Input: part model. Units: mm. Frame: model coordinates. Face numbers are marked on the shaded views. A direction names the side the tool comes from. Give positions to 0.01 mm unless a question says otherwise; leave off trailing zeros. Loops run counter-clockwise (first coordinate to the right, second up) from the corner with the lowest first, then second, coordinate; pieces in that order, holes last. Notation, with made-up numbers: (77.25, 62) -> (111.25, 62) arc R17 cw to (111.25, 82) -> close; hole circle Ø9 at (53, 76.25). An arc over 180 degrees is marked (long way). One line per question, with ' | ' between items.
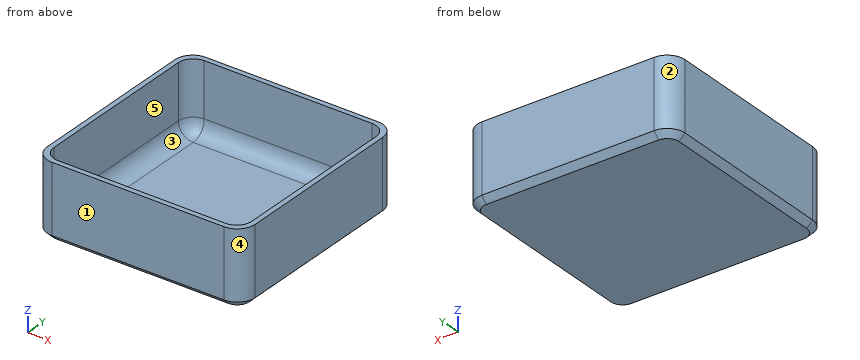
from build123d import *

# Parameters (mm, degrees)
F0_W     = 70
F0_H     = 70
F0_W_2   = 66.6
F0_H_2   = 66.6
F1_DEPTH = 25
F2_W     = 66.6
F2_H     = 66.6
F3_DEPTH = 23.3
F4_R     = 5
F5_R     = 6
F6_SIZE  = 2


with BuildPart() as f1:
    # F0 (on Top) → F1 (new body)
    with BuildSketch(Plane.XY):
        Rectangle(F0_W, F0_H)
        Rectangle(F0_W_2, F0_H_2, mode=Mode.SUBTRACT)
        Rectangle(F0_W_2, F0_H_2)
    extrude(amount=F1_DEPTH)

    # F2 (on face) → F3 (cut)
    with BuildSketch(Plane.XY.offset(25)):
        Rectangle(F2_W, F2_H)
    extrude(amount=-F3_DEPTH, mode=Mode.SUBTRACT)

    # F4
    f4_edges = [f1.edges().sort_by_distance(p)[0] for p in [
        (-33.3, 0, 1.7),
        (33.3, 0, 1.7),
        (-33.3, 33.3, 13.35),
        (0, 33.3, 1.7),
        (-33.3, -33.3, 13.35),
        (0, -33.3, 1.7),
        (33.3, -33.3, 13.35),
        (33.3, 33.3, 13.35),
    ]]
    fillet(f4_edges, radius=F4_R)

    # F5
    f5_edges = [f1.edges().sort_by_distance(p)[0] for p in [
        (35, 35, 12.5),
        (-35, 35, 12.5),
        (35, -35, 12.5),
        (-35, -35, 12.5),
    ]]
    fillet(f5_edges, radius=F5_R)

    # F6
    f6_edges = [f1.edges().sort_by_distance(p)[0] for p in [
        (35, 0, 0),
    ]]
    chamfer(f6_edges, length=F6_SIZE)


solid = f1.part
1. Section query A-A (z = 9.25). Output: boundary loops of the cut face in (x, y).
Determined:
outline: (-35, -29) arc R6 ccw to (-29, -35) -> (29, -35) arc R6 ccw to (35, -29) -> (35, 29) arc R6 ccw to (29, 35) -> (-29, 35) arc R6 ccw to (-35, 29) -> close; hole (-33.3, -28.3) arc R5 ccw to (-28.3, -33.3) -> (28.3, -33.3) arc R5 ccw to (33.3, -28.3) -> (33.3, 28.3) arc R5 ccw to (28.3, 33.3) -> (-28.3, 33.3) arc R5 ccw to (-33.3, 28.3) -> close
2. Reachability of the marked faces 4 and 5 from +Z, -Z, +X, -X, +Y, -Y: full face, straight path, thin tool, end or side. Return the list, or none.
Determined:
face 4: +Z, -Z, +X, -Y | face 5: +Z
3. Section query B-B (y = -21). Output: boundary loops of the cut face in (x, z).
Determined:
outline: (-35, 2) -> (-33, 0) -> (33, 0) -> (35, 2) -> (35, 25) -> (33.3, 25) -> (33.3, 6.7) arc R5 cw to (28.3, 1.7) -> (-28.3, 1.7) arc R5 cw to (-33.3, 6.7) -> (-33.3, 25) -> (-35, 25) -> close
4. Section query D-D (z = 4). Output: boundary loops of the cut face in (x, y).
Determined:
outline: (-35, -29) arc R6 ccw to (-29, -35) -> (29, -35) arc R6 ccw to (35, -29) -> (35, 29) arc R6 ccw to (29, 35) -> (-29, 35) arc R6 ccw to (-35, 29) -> close; hole (-32.51, -28.3) arc R4.21 ccw to (-28.3, -32.51) -> (28.3, -32.51) arc R4.21 ccw to (32.51, -28.3) -> (32.51, 28.3) arc R4.21 ccw to (28.3, 32.51) -> (-28.3, 32.51) arc R4.21 ccw to (-32.51, 28.3) -> close
5. Pull-direction query (X, two-part tool) for the marked faces 1, 2 and 3; classes: pulls with the +X half, pulls with the -X half, needs draft (parallel to the pull), parting line crosses it, or undercut.
Determined:
face 1: needs draft | face 2: pulls with the -X half | face 3: undercut
6. Ray query, line 1 along Y through (x, z) = (-18, 22); line 2 along Y through (x, z) = (8.5, 5). Return the intervals inside material, ascending. Write a range as from..to.
Determined:
line 1: y = -35..-33.3, 33.3..35 | line 2: y = -35..-33, 33..35
